Geometry check sheet. Reference: the model listing, model coordinates, mm. A direction names the side the tool comes from. Round coordinates to 2 decimals unless told otherwise and drop trailing zeros. Write each loop counter-clockwise with the first axis right and the second up, starting at its lowest first coordinate (ties: lowest second). Pieces come first, ordered by that corner, then holes. Notation, with made-up numbers: (-14.5, 51.5) - (8.5, 51.5) arc R36 ccw to (8.5, 89.5) - close; hole circle Ø7 at (73, -34). An arc over 180 degrees is marked (long way). Return JSON: item names as keys, results as strings.
```python
from build123d import *

# Parameters (mm, degrees)
F0_R     = 3.25
F0_R_2   = 1
F1_DEPTH = 5
F2_DEPTH = 3
F3_W     = 6.5
F3_H     = 0.8
F4_DEPTH = 25


with BuildPart() as f1:
    # F0 (on Top) → F1 (new body)
    with BuildSketch(Plane.XY):
        with BuildLine():
            ThreePointArc((-7.9180477187, -2.6999995224), (-5.2663972893, -1.6016499519), (-4.1680477187, 1.0500004776))
            ThreePointArc((-4.1680477187, 1.0500004776), (-4.1701339523, 1.1750700574), (-4.1763903319, 1.3000004776))
            ThreePointArc((-4.1763903319, 1.3000004776), (-4.2448197056, 1.8049150184), (-4.3810640575, 2.2958923592))
            ThreePointArc((-4.3810640575, 2.2958923592), (-10.9786517895, 3.2168421243), (-7.9180477187, -2.6999995224))
        make_face()
        with Locations((-7.9180477187, 1.0500004776)):
            Circle(F0_R, mode=Mode.SUBTRACT)
        with Locations((-7.9180477187, 1.0500004776)):
            Circle(F0_R)
        with Locations((-7.9180477187, 1.0500004776)):
            Circle(F0_R_2, mode=Mode.SUBTRACT)
        with BuildLine():
            ThreePointArc((6.3404704502, 1.3000004776), (7.3435150495, -1.5117372139), (10.082127837, -2.6999995224))
            ThreePointArc((10.082127837, -2.6999995224), (12.7337782665, -1.6016499519), (13.832127837, 1.0500004776))
            ThreePointArc((13.832127837, 1.0500004776), (10.7141133078, 4.7463627927), (6.5451441758, 2.2958923592))
            ThreePointArc((6.5451441758, 2.2958923592), (6.4088998239, 1.8049150184), (6.3404704502, 1.3000004776))
        make_face()
        with Locations((10.082127837, 1.0500004776)):
            Circle(F0_R, mode=Mode.SUBTRACT)
        with Locations((10.082127837, 1.0500004776)):
            Circle(F0_R)
        with Locations((10.082127837, 1.0500004776)):
            Circle(F0_R_2, mode=Mode.SUBTRACT)
        with BuildLine():
            ThreePointArc((-4.1763903319, 1.3000004776), (-4.1701339523, 1.1750700574), (-4.1680477187, 1.0500004776))
            ThreePointArc((-4.1680477187, 1.0500004776), (-5.2663972893, -1.6016499519), (-7.9180477187, -2.6999995224))
            Line((-7.9180477187, -2.6999995224), (10.082127837, -2.6999995224))
            ThreePointArc((10.082127837, -2.6999995224), (7.3435150495, -1.5117372139), (6.3404704502, 1.3000004776))
            Line((6.3404704502, 1.3000004776), (5.2561087846, 1.3000004776))
            Line((5.2561087846, 1.3000004776), (-3.0920286663, 1.3000004776))
            Line((-3.0920286663, 1.3000004776), (-4.1763903319, 1.3000004776))
        make_face()
        with BuildLine():
            ThreePointArc((-4.3810640575, 2.2958923592), (-4.2448197056, 1.8049150184), (-4.1763903319, 1.3000004776))
            Line((-4.1763903319, 1.3000004776), (-3.0920286663, 1.3000004776))
            ThreePointArc((-3.0920286663, 1.3000004776), (-3.8704928802, 1.6245723747), (-4.3810640575, 2.2958923592))
        make_face()
        with BuildLine():
            ThreePointArc((6.5451441758, 2.2958923592), (6.0345729985, 1.6245723747), (5.2561087846, 1.3000004776))
            Line((5.2561087846, 1.3000004776), (6.3404704502, 1.3000004776))
            ThreePointArc((6.3404704502, 1.3000004776), (6.4088998239, 1.8049150184), (6.5451441758, 2.2958923592))
        make_face()
    extrude(amount=F1_DEPTH)

    # F0 (on Top) → F2 (cut)
    with BuildSketch(Plane.XY):
        with Locations((10.082127837, 1.0500004776)):
            Circle(F0_R)
        with Locations((10.082127837, 1.0500004776)):
            Circle(F0_R_2, mode=Mode.SUBTRACT)
        with Locations((-7.9180477187, 1.0500004776)):
            Circle(F0_R)
        with Locations((-7.9180477187, 1.0500004776)):
            Circle(F0_R_2, mode=Mode.SUBTRACT)
    extrude(amount=F2_DEPTH, mode=Mode.SUBTRACT)

    # F3 (on face) → F4 (cut)
    with BuildSketch(Plane.XZ.offset(2.6999995224)):
        with Locations((1.0820400592, 2.5)):
            Rectangle(F3_W, F3_H)
    extrude(amount=-F4_DEPTH, mode=Mode.SUBTRACT)


solid = f1.part
```
(1) Section check D-D, the plane x = 7.75. Enter the section's corners in (y, z), plus the area to 3 significant figures.
Response values:
{"outline": "(-2.7, 0) - (-1.21, 0) - (-1.21, 3) - (3.31, 3) - (3.31, 0) - (3.99, 0) - (3.99, 5) - (-2.7, 5) - close", "area": "19.9 mm^2"}
(2) Material ranges on line 1 along X through (y, z) = (0.5, 2.8); line 2 along Z through (x, y) = (3, 1.25); line 3 along X through (y, z) = (4, 2.25), recorded low to high. Write a range as [from, to].
Response values:
{"line 1": "x = [-11.63, -11.12], [-4.71, -2.17], [4.33, 6.88], [13.29, 13.79]", "line 2": "z = [0, 2.1], [2.9, 5]", "line 3": "x = [-10.23, -9.28], [-6.55, -5.6], [7.77, 8.72], [11.45, 12.4]"}
(3) Release check for a two-part mould opening along Y. For faces 1 (the face through (9.083, 1.094, 3.986)), 2 (the face through (1, 0, 5)), 3 (the face through (1, -2.7, 1.9)) record: pulls with the +Y half, pulls with the -Y half, needs draft (parallel to the pull), parting line crosses it, or undercut.
Response values:
{"face 1": "undercut", "face 2": "needs draft", "face 3": "pulls with the -Y half"}
(4) Section check C-C, the plane z = 3.65. Enter the section's corners in (x, y).
Response values:
{"outline": "(-7.92, -2.7) - (10.08, -2.7) arc R3.75 ccw (long way) to (6.55, 2.3) arc R1.62 cw to (5.26, 1.3) - (-3.09, 1.3) arc R1.62 cw to (-4.38, 2.3) arc R3.75 ccw (long way) to start; hole circle Ø2 at (-7.92, 1.05); hole circle Ø2 at (10.08, 1.05)"}
(5) Section check A-A, the plane z = 2.55. Enter the section's corners in (x, y), plus the area to 3 significant figures.
Response values:
{"outline": "(-7.92, -2.7) - (-2.17, -2.7) - (-2.17, 1.3) - (-3.09, 1.3) arc R1.62 cw to (-4.38, 2.3) arc R3.75 ccw (long way) to start; (4.33, -2.7) - (10.08, -2.7) arc R3.75 ccw (long way) to (6.55, 2.3) arc R1.62 cw to (5.26, 1.3) - (4.33, 1.3) - close; hole circle Ø6.5 at (-7.92, 1.05); hole circle Ø6.5 at (10.08, 1.05)", "area": "44.6 mm^2"}
(6) Access from +Z, -Z, +X, -X, +Y, -Y to the whole of each face (thin tool, end or side, straight path). Record for faces 4 (the face through (4.332, -0.7, 2.5)), 5 (the face through (-10.91, 3.31, 2.46)), 6 (the face through (1, 0, 0)), 7 (the face through (-3.861, 1.617, 2.465)), 8 (the face through (-11.165, 1.193, 1.479)).
Response values:
{"face 4": "+Y, -Y", "face 5": "+Z, -Z", "face 6": "-Z, +X, -X, +Y, -Y", "face 7": "+Z, -Z, +Y", "face 8": "-Z"}
(7) Section check B-B, the plane x = 2.75. Enter the section's corners in (y, z).
Response values:
{"outline": "(-2.7, 0) - (1.3, 0) - (1.3, 2.1) - (-2.7, 2.1) - close; (-2.7, 2.9) - (1.3, 2.9) - (1.3, 5) - (-2.7, 5) - close"}
(8) Gauge pin test, flat ends, axial feed: pin 1 (1.5 mm diameter, centred on x = 1.5, z = 1.5, fed in from +Y); pin 2 (3 mm diameter, centred on x = 10, y = 1, fed in from -Z). Record the tip position at first contact, or that the pin passes through.
Response values:
{"pin 1": "stops at y = 1.3", "pin 2": "stops at z = 3"}
